Verification items for the finished model (mm, model axes). Coordinates: 2 decimals unless noted, no trailing zeros. Loops run counter-clockwise (first coordinate to the right, second up) from the corner with the lowest first, then second, coordinate; pieces in that order, holes last. Notation, with made-up numbers: (4, 9) - (59, 9) arc R12 cw to (59, 30) - close; hole circle Ø5 at (69, 69.5). An arc over 180 degrees is marked (long way). One line per item, written item: value. Start each with the question number.
(1) Section check B-B (z = 9). Record the boundary of the cut face in (x, y), plus the area to 3 significant figures.
(2) Section check A-A (y = 0). Record the boundary of the cut face in (x, z).
(3) Draft check along Y on faces 1 (the face through (-108.834, -6.703, 9.86)), 2 (the face through (159.964, 45.742, 10.07)), 3 (the face through (-175, -25, 10)). Enter one of: +Y half, -Y half, draft (parallel to the pull), parting line (faces both ways), or undercut.
(4) Section check C-C (x = 119). Record the boundary of the cut face in (y, z).
(5) Thickness scan on probe 1 along Y at (x, z) = (-125, 11.25); probe 2 along Y at (x, z) = (-153.5, 11.25); probe 3 along X at (y, z) = (52, 4.75). Record the ranges inside material, lowest first. Write a range as [from, to].
(6) Gauge pin test, flat ends, axial feed: P1, Ø8, axis at y = 19, z = 11, coming from the +X side; P2, Ø21, axis at x = 125, y = 0, coming from the -Z side; P3, Ø5, axis at y = -2.5, z = 18, coming from the -X side; P4, Ø1, axis at y = 9.5, z = 16, coming from the +X side. Record the tip position at first contact, or that the pin passes through.
```python
from build123d import *

# Parameters (mm, degrees)
F0_W     = 350
F0_H     = 120
F0_R     = 17.5
F1_DEPTH = 20
F2_R     = 50
F3_SIZE  = 5


with BuildPart() as f1:
    # F0 (on Top) → F1 (new body)
    with BuildSketch(Plane.XY):
        Rectangle(F0_W, F0_H)
        with Locations((-125, 0)):
            Circle(F0_R, mode=Mode.SUBTRACT)
        with Locations((125, 0)):
            Circle(F0_R, mode=Mode.SUBTRACT)
    extrude(amount=F1_DEPTH)

    # F2
    f2_edges = [f1.edges().sort_by_distance(p)[0] for p in [
        (175, 60, 10),
        (-175, 60, 10),
    ]]
    fillet(f2_edges, radius=F2_R)

    # F3
    f3_edges = [f1.edges().sort_by_distance(p)[0] for p in [
        (175, -25, 0),
        (0, 60, 20),
    ]]
    chamfer(f3_edges, length=F3_SIZE)


solid = f1.part
```
Responses:
1. outline: (-175, -60) - (175, -60) - (175, 10) arc R50 ccw to (125, 60) - (-125, 60) arc R50 ccw to (-175, 10) - close; hole circle Ø35 at (-125, 0); hole circle Ø35 at (125, 0)
1. area: 39,000 mm²
2. outline: (-175, 5) - (-170, 0) - (-142.5, 0) - (-142.5, 20) - (-170, 20) - (-175, 15) - close; (-107.5, 0) - (107.5, 0) - (107.5, 20) - (-107.5, 20) - close; (142.5, 0) - (170, 0) - (175, 5) - (175, 15) - (170, 20) - (142.5, 20) - close
3. face 1: undercut
3. face 2: +Y half
3. face 3: draft
4. outline: (-60, 0) - (-16.44, 0) - (-16.44, 20) - (-60, 20) - close; (16.44, 0) - (55, 0) - (60, 5) - (60, 15) - (55, 20) - (16.44, 20) - close
5. probe 1: y = [-60, -17.5], [17.5, 60]
5. probe 2: y = [-60, 51.08]
5. probe 3: x = [-151.67, 151.67]
6. P1: stops at x = 174.75
6. P2: passes through
6. P3: stops at x = -174.5
6. P4: stops at x = 174.5
